Part model, mm, in its own coordinate system. Face numbers are marked on the shaded views. A direction names the side the tool comes from. Round coordinates to 2 decimals unless told otherwise and drop trailing zeros. Loops run counter-clockwise (first coordinate to the right, second up) from the corner with the lowest first, then second, coordinate; pieces in that order, holes last. Notation, with made-up numbers: M 17,70 L 66,70 A26 cw 66,100 Z; hole C 59,39.25 d2. An arc over 180 degrees is marked long. Answer as CSV lines item,"result". Start each with the question number.
Item 1: Wall check: line 1 (Z direction, x = 0, y = 0.9) (3 decimals); line 2 (Y direction, x = 2, z = -5.5); line 3 (Z direction, x = 0, y = 4.15) (3 decimals). Give the ranges that are in metal, low to high.
Item 2: Band-saw the part on B-B (x = 0). Count the separate pieces of the cut face and the enclosed holes in it, and give its area (3 significant figures).
Item 3: Drop flat-ended pins along their axis: pin 1 Ø1.5 at (x, z) = (-1, 1) entering from -Y; pin 2 Ø2 at (y, z) = (1.5, 3) entering from +X; pin 3 Ø6 at (x, z) = (5, -7) entering from +Y. Give the stop position or say it passes through.
Item 4: Mould opens along Z. For the marked faces 4, 5, 6 and 7 say: pulls with the +Z half, pulls with the -Z half, needs draft (parallel to the pull), parting line crosses it, or undercut.
Item 5: Which spindle directions (+Z, -Z, +X, -X, +Y, -Y) get a long thin tool onto all of the face, cutting with end or side? Do the marked faces 1, 2 and 3. Say none if no direction does.
Item 6: Band-saw the part on A-A (y = 1.2). Give the cut face in (x, z) (3 decimals), and give its area (3 significant figures).
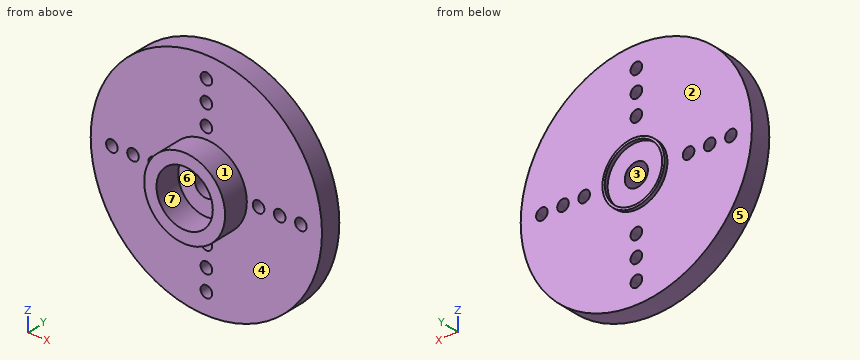
```python
from build123d import *

# Parameters (mm, degrees)
SKETCH2_R           = 2.685
SKETCH2_R_2         = 2.485
BOSS_EXTRUDE1_DEPTH = 0.3
SKETCH4_R           = 0.5
CUT_EXTRUDE2_DEPTH  = 5.36
CIRPATTERN1_COUNT   = 4


with BuildPart() as part:
    # Sketch1 → Revolve2 (revolve)
    with BuildSketch(Plane.XY):
        Polygon((1, 2.26), (1, 4.06), (10, 4.06), (10, 2.26), (3.5, 2.26), (3.5, 0), (2.435, 0), (2.435, 2.26), align=None)
    revolve(axis=Axis((0, 0, 0), (0, 1, 0)))

    # Sketch2 → Boss-Extrude1 (add)
    with BuildSketch(Plane(origin=(0, 4.06, 0), x_dir=(1, 0, 0), z_dir=(0, 1, 0))):
        Circle(SKETCH2_R)
        Circle(SKETCH2_R_2, mode=Mode.SUBTRACT)
    extrude(amount=BOSS_EXTRUDE1_DEPTH)

    # Sketch4 → Cut-Extrude2 (cut, through all)
    with BuildSketch(Plane(origin=(0, 0, 0), x_dir=(1, 0, 0), z_dir=(0, 1, 0))):
        with Locations((0, 4.51375)):
            Circle(SKETCH4_R)
        with Locations((0, 6.3425)):
            Circle(SKETCH4_R)
        with Locations((0, 8.17125)):
            Circle(SKETCH4_R)
    cut_extrude2 = extrude(amount=CUT_EXTRUDE2_DEPTH, mode=Mode.SUBTRACT)

    # CirPattern1: Cut-Extrude2 ×4 about axis
    cirpattern1_axis = Axis((0, 0, 0), (0, 1, 0))
    for i in range(1, CIRPATTERN1_COUNT):
        add(cut_extrude2.rotate(cirpattern1_axis, i * 360 / CIRPATTERN1_COUNT), mode=Mode.SUBTRACT)


solid = part.part
```
Answer block:
1,line 1,"z = -3.5 to -2.435, 2.435 to 3.5"
1,line 2,"y = 2.26 to 4.06"
1,line 3,"z = -2.685 to -2.485, 2.485 to 2.685"
2,separate pieces,"8"
2,enclosed holes,"0"
2,area,"26.5 mm^2"
3,pin 1,"stops at y = 2.26"
3,pin 2,"stops at x = 9.72"
3,pin 3,"stops at y = 4.06"
4,face 4,"needs draft"
4,face 5,"parting line crosses it"
4,face 6,"undercut"
4,face 7,"undercut"
5,face 1,"-Y"
5,face 2,"+Y"
5,face 3,"+Y, -Y"
6,outline,"C 0,0 d7; hole C 0,0 d4.87"
6,area,"19.9 mm^2"
